from build123d import *

# Parameters (mm, degrees)
F0_W          = 7.62
F0_H          = 25.4
F1_DEPTH      = 25.4
F5_R          = 10.922
F6_DEPTH      = 6.985
F4_R          = 6.985
F4_R_2        = 3.81
F7_DEPTH      = 3.175
F7_DEPTH_BACK = 3.175
F8_DEPTH      = 10.16
F8_DEPTH_BACK = 3.175
F9_R          = 5.08
F10_R         = 2.54


# Not quite as in the source:
# - a pattern or mirror of a feature is missing from the dataset's text; its kind, count and spacing are read off the source's solid


with BuildPart() as f1:
    # F0 (on Top) → F1 (new body)
    with BuildSketch(Plane.XY):
        with BuildLine():
            Line((55.245, 0), (47.625, 0))
            ThreePointArc((47.625, 0), (0, -47.625), (-47.625, 0))
            Line((-47.625, 0), (-55.245, 0))
            ThreePointArc((-55.245, 0), (0, -55.245), (55.245, 0))
        make_face()
        with Locations((51.435, 12.7)):
            Rectangle(F0_W, F0_H)
        with Locations((-51.435, 12.7)):
            Rectangle(F0_W, F0_H)
    extrude(amount=F1_DEPTH)

    # F5 (on face) → F6 (cut)
    with BuildSketch(Plane(origin=(47.625, 0, 0), x_dir=(0, -1, 0), z_dir=(-1, 0, 0))):
        with Locations((-12.7, 12.7)):
            Circle(F5_R)
    f6 = extrude(amount=-F6_DEPTH, mode=Mode.SUBTRACT)

    # F6_copies: F6 across plane
    add(f6.mirror(Plane(origin=(0, 0, 0), x_dir=(0, 0, -1), z_dir=(-1, 0, 0))), mode=Mode.SUBTRACT)

    # F4 (on plane+point) → F7 (join, two sides)
    with BuildSketch(Plane.XZ.offset(55.245)) as f7_sk:
        with Locations((0, 12.7)):
            Circle(F4_R)
        with Locations((0, 12.7)):
            Circle(F4_R_2, mode=Mode.SUBTRACT)
    extrude(amount=F7_DEPTH)
    extrude(f7_sk.sketch, amount=-F7_DEPTH_BACK)

    # F4 (on plane+point) → F8 (join, two sides)
    with BuildSketch(Plane.XZ.offset(55.245)) as f8_sk:
        with Locations((0, 12.7)):
            Circle(F4_R_2)
    extrude(amount=F8_DEPTH)
    extrude(f8_sk.sketch, amount=-F8_DEPTH_BACK)

    # F9
    f9_edges = [f1.edges().sort_by_distance(p)[0] for p in [
        (-51.435, 25.4, 0),
        (-51.435, 25.4, 25.4),
        (51.435, 25.4, 25.4),
        (51.435, 25.4, 0),
    ]]
    fillet(f9_edges, radius=F9_R)

    # F10
    f10_edges = [f1.edges().sort_by_distance(p)[0] for p in [
        (0, -55.245, 0),
        (55.245, 25.4, 12.7),
        (55.245, 23.912102, 1.487898),
        (55.245, 23.912102, 23.912102),
        (-55.245, 10.16, 0),
        (55.245, 10.16, 0),
        (-55.245, 10.16, 25.4),
        (0, -55.245, 25.4),
        (55.245, 10.16, 25.4),
        (-55.245, 23.912102, 1.487898),
        (-55.245, 25.4, 12.7),
        (-55.245, 23.912102, 23.912102),
    ]]
    fillet(f10_edges, radius=F10_R)


solid = f1.part
Design review of the part built by this model. Coordinates are the model's own, in mm. A direction names the side the tool comes from. Coordinates: 2 decimals unless noted, no trailing zeros. Write each loop counter-clockwise with the first axis right and the second up, starting at its lowest first coordinate (ties: lowest second). Pieces come first, ordered by that corner, then holes. Notation, with made-up numbers: (31, 2.5) - (63, 2.5) arc R12 cw to (63, 25.5) - close; hole circle Ø6 at (5, 0). An arc over 180 degrees is marked (long way). Use one line per item in the form item = value.
Q1. For probe 1 along X at (y, z) = (9.5, 21.5) (3 decimals); probe 2 along X at (y, z) = (0.5, 11) (3 decimals); probe 3 along Z at (x, y) = (51, 12), list the stretches that pass through material, from the lowest coordinate up.
Taken from the geometry:
probe_1 = -55.245 to -54.61, 54.61 to 55.245
probe_2 = -55.245 to -47.625, 47.625 to 55.245
probe_3 = 0 to 1.8, 23.6 to 25.4
Q2. Consider section C-C (z = 12.7). Write out the cut boundary in (x, y) (3 decimals), plus the area to 3 significant figures.
Taken from the geometry:
outline = (-55.245, 0) arc R55.245 ccw to (-6.985, -54.802) - (-6.985, -58.42) - (-3.81, -58.42) - (-3.81, -65.405) - (3.81, -65.405) - (3.81, -58.42) - (6.985, -58.42) - (6.985, -54.802) arc R55.245 ccw to (55.245, 0) - (55.245, 22.86) arc R2.54 ccw to (52.705, 25.4) - (47.625, 25.4) - (47.625, 23.622) - (54.61, 23.622) - (54.61, 1.778) - (47.625, 1.778) - (47.625, 0) arc R47.625 cw to (-47.625, 0) - (-47.625, 1.778) - (-54.61, 1.778) - (-54.61, 23.622) - (-47.625, 23.622) - (-47.625, 25.4) - (-52.705, 25.4) arc R2.54 ccw to (-55.245, 22.86) - close
area = 1,410 mm^2
Q3. Consider section A-A (y = 12.7). Write out the cut boundary in (x, z) (3 decimals), plus the area to 3 significant figures.
Taken from the geometry:
outline = (-55.245, 2.54) arc R2.54 ccw to (-52.705, 0) - (-47.625, 0) - (-47.625, 1.778) - (-54.61, 1.778) - (-54.61, 23.622) - (-47.625, 23.622) - (-47.625, 25.4) - (-52.705, 25.4) arc R2.54 ccw to (-55.245, 22.86) - close; (47.625, 0) - (52.705, 0) arc R2.54 ccw to (55.245, 2.54) - (55.245, 22.86) arc R2.54 ccw to (52.705, 25.4) - (47.625, 25.4) - (47.625, 23.622) - (54.61, 23.622) - (54.61, 1.778) - (47.625, 1.778) - close
area = 76.4 mm^2
Q4. Machinability: for faces 4 (the flat face through (-50, 25.4, 13)), 5 (the flat face through (-54.61, 13, 13)), 6 (the flat face through (47.625, 13, 24)), which of the approach directions +Z, -Z, +X, -X, +Y, -Y give a long, thin tool a straight path to every point of the face, cutting with its end or side? Answer none if there is none.
Taken from the geometry:
face_4 = +Z, -Z, +X, -X, +Y
face_5 = none
face_6 = +Z, -Z, +Y
Q5. Insertion check: pin 1 Ø8 at (x, y) = (39, -44) entering from -Z; pin 2 Ø6 at (x, z) = (7.5, 5.5) entering from -Y; pin 3 Ø10 at (y, z) = (-30.5, 7) entering from -X. Each pin has a flat end and moves straight along its axis. Give the tip position at first contact, or say it passes through.
Taken from the geometry:
pin_1 = 1.1
pin_2 = -55.06
pin_3 = -49.01
Q6. Consider section B-B (x = 0). Write out the cut boundary in (y, z) (3 decimals).
Taken from the geometry:
outline = (-65.405, 8.89) - (-58.42, 8.89) - (-58.42, 5.715) - (-55.245, 5.715) - (-55.245, 2.54) arc R2.54 ccw to (-52.705, 0) - (-47.625, 0) - (-47.625, 25.4) - (-52.705, 25.4) arc R2.54 ccw to (-55.245, 22.86) - (-55.245, 19.685) - (-58.42, 19.685) - (-58.42, 16.51) - (-65.405, 16.51) - close
Q7. The part is to be moulded in two halves that separate along Y. For faces 1 (the cylindrical face through (-54.481, 10.018, 0.724)), 2 (the cylindrical face through (50.201, 23.872, 23.951)), 3 (the cylindrical face through (51.07, 2.61, 8.52)), say which applies: +Y half, -Y half, draft (parallel to the pull), parting line (faces both ways), or undercut.
Taken from the geometry:
face_1 = draft
face_2 = +Y half
face_3 = undercut
